```python
from build123d import *

# Parameters (mm, degrees)
SKETCH_1_R      = 15
SKETCH_1_R_2    = 1.3
SKETCH_1_R_3    = 0.7
EXTRUDE_2_DEPTH = 1.4
SKETCH_2_W      = 5.5
SKETCH_2_H      = 5.5
SKETCH_2_W_2    = 10.16
SKETCH_2_H_2    = 3.68
EXTRUDE_5_DEPTH = 1.5
SKETCH_3_W      = 5
SKETCH_3_H      = 3.37
EXTRUDE_7_DEPTH = 1.5


with BuildPart() as part:
    # 草图1 → 凸台-拉伸2 (new body)
    with BuildSketch(Plane(origin=(0, 0, 0), x_dir=(1, 0, 0), z_dir=(0, 1, 0))):
        with Locations(Location((0, 0, 0), (0, 0, 270))):
            Circle(SKETCH_1_R)
        with Locations(Location((-7.778174593, 7.778174593, 0), (0, 0, 270))):
            Circle(SKETCH_1_R_2, mode=Mode.SUBTRACT)
        with Locations(Location((7.778174593, 7.778174593, 0), (0, 0, 270))):
            Circle(SKETCH_1_R_2, mode=Mode.SUBTRACT)
        with Locations(Location((7.778174593, -7.778174593, 0), (0, 0, 270))):
            Circle(SKETCH_1_R_2, mode=Mode.SUBTRACT)
        with Locations(Location((-7.778174593, -7.778174593, 0), (0, 0, 270))):
            Circle(SKETCH_1_R_2, mode=Mode.SUBTRACT)
        with Locations(Location((-3.81, 12.8, 0), (0, 0, 270))):
            Circle(SKETCH_1_R_3, mode=Mode.SUBTRACT)
        with Locations(Location((-1.27, 12.8, 0), (0, 0, 270))):
            Circle(SKETCH_1_R_3, mode=Mode.SUBTRACT)
        with Locations(Location((1.27, 12.8, 0), (0, 0, 270))):
            Circle(SKETCH_1_R_3, mode=Mode.SUBTRACT)
        with Locations(Location((3.81, 12.8, 0), (0, 0, 270))):
            Circle(SKETCH_1_R_3, mode=Mode.SUBTRACT)
    extrude(amount=EXTRUDE_2_DEPTH)

    # 草图2 → 凸台-拉伸5 (add)
    with BuildSketch(Plane(origin=(0, 1.4, 0), x_dir=(1, 0, 0), z_dir=(0, 1, 0))):
        Rectangle(SKETCH_2_W, SKETCH_2_H)
        with Locations((-1.15, -9.46)):
            Rectangle(SKETCH_2_W_2, SKETCH_2_H_2)
    extrude(amount=EXTRUDE_5_DEPTH)

    # 草图3 → 凸台-拉伸7 (add)
    with BuildSketch(Plane.XZ):
        Rectangle(SKETCH_3_W, SKETCH_3_H)
    extrude(amount=EXTRUDE_7_DEPTH)


solid = part.part
```
Model file for the job. Use its own axes, mm. A direction names the side the tool comes from. Coordinates: 2 decimals unless noted, no trailing zeros. Order: outer loops, then holes, each group sorted by start corner. A loop starts at its lowest first (then second) coordinate and runs counter-clockwise, first axis right, second up. Notation, with made-up numbers: (-28.5, 41) -> (-4.5, 41) arc R13 ccw to (-4.5, 49) -> close; hole circle Ø11 at (16, 44). An arc over 180 degrees is marked (long way). Answer as a JSON object with one key per item and string values. Group by question number.
1) Drill centre lines: L1, parallel to Z at x = 0.25, y = 2.3; L2, parallel to Z at x = -7.5, y = 1.15; L3, parallel to Y at x = 3.5, z = -5.25. Where is each one in solid material? Low to high.
2) Cut at B-B, the plane x = -3.81. Write the cut outline in (y, z), then the cut area to 3 significant figures.
3) Which spindle directions (+Z, -Z, +X, -X, +Y, -Y) get a long thin tool onto all of the face, cutting with end or side? Do faces 1 (the face through (-2.75, 2, 0)), 2 (the face through (-2.5, -1, 0)), 3 (the face through (2.75, 2, 0)), 4 (the face through (0, -1, -1.685)). Say none if no direction does.
4) Cut at D-D, the plane x = 0. Write the cut outline in (y, z) (3 decimals), then the cut area to 3 significant figures.
5) Cut at C-C, the plane z = -12.8. Write the cut outline in (x, y), then the cut area to 3 significant figures.
6) Cut at A-A, the plane y = 2.05. Write the cut outline in (x, z), then the cut area to 3 significant figures.
7) Pull direction X, two halves, no side cores. Call faces 5 (the face through (2.5, -1, 0)), 6 (the face through (-1.538, 0.69, -12.153)), 7 (the face through (0, 2, -2.75)), 8 (the face through (-3.6, 0.69, -12.132)): +X half, -X half, draft (parallel to the pull), parting line (faces both ways), or undercut.
8) Flat gauge pins, fed straight in: pin 1 (1.5 mm diameter, centred on x = -1.5, y = 2.5, fed in from -Z); pin 2 (2.5 mm diameter, centred on x = -7.78, z = 7.78, fed in from -Y); pin 3 (1.2 mm diameter, centred on y = -1, z = -0.5, fed in from +X); pin 4 (1.8 mm diameter, centred on x = 1.27, z = -12.8, fed in from -Y). Where does each tip first touch, or does it go through?
Check values:
{
 "1": {"L1": "z = -2.75 to 2.75, 7.62 to 11.3", "L2": "z = -12.99 to -9.05, -6.51 to 6.51, 9.05 to 12.99", "L3": "y = 0 to 1.4"},
 "2": {"outline": "(0, -14.51) -> (1.4, -14.51) -> (1.4, -13.5) -> (0, -13.5) -> close; (0, -12.1) -> (1.4, -12.1) -> (1.4, 7.62) -> (2.9, 7.62) -> (2.9, 11.3) -> (1.4, 11.3) -> (1.4, 14.51) -> (0, 14.51) -> close", "area": "44.2 mm²"},
 "3": {"face 1": "-Z, -X, +Y", "face 2": "+Z, -Z, -X, -Y", "face 3": "-Z, +X, +Y", "face 4": "-Z, +X, -X, -Y"},
 "4": {"outline": "(-1.5, -1.685) -> (0, -1.685) -> (0, -15) -> (1.4, -15) -> (1.4, -2.75) -> (2.9, -2.75) -> (2.9, 2.75) -> (1.4, 2.75) -> (1.4, 7.62) -> (2.9, 7.62) -> (2.9, 11.3) -> (1.4, 11.3) -> (1.4, 15) -> (0, 15) -> (0, 1.685) -> (-1.5, 1.685) -> close", "area": "60.8 mm²"},
 "5": {"outline": "(-7.82, 0) -> (-4.51, 0) -> (-4.51, 1.4) -> (-7.82, 1.4) -> close; (-3.11, 0) -> (-1.97, 0) -> (-1.97, 1.4) -> (-3.11, 1.4) -> close; (-0.57, 0) -> (0.57, 0) -> (0.57, 1.4) -> (-0.57, 1.4) -> close; (1.97, 0) -> (3.11, 0) -> (3.11, 1.4) -> (1.97, 1.4) -> close; (4.51, 0) -> (7.82, 0) -> (7.82, 1.4) -> (4.51, 1.4) -> close", "area": "14.1 mm²"},
 "6": {"outline": "(-6.23, 7.62) -> (3.93, 7.62) -> (3.93, 11.3) -> (-6.23, 11.3) -> close; (-2.75, -2.75) -> (2.75, -2.75) -> (2.75, 2.75) -> (-2.75, 2.75) -> close", "area": "67.6 mm²"},
 "7": {"face 5": "+X half", "face 6": "undercut", "face 7": "draft", "face 8": "undercut"},
 "8": {"pin 1": "stops at z = -2.75", "pin 2": "passes through", "pin 3": "stops at x = 2.5", "pin 4": "stops at y = 0"}
}
